from build123d import *

# Parameters (mm, degrees)
CROSSRECESS_DEPTH = 2.17
FILLET5_R         = 0.3
DRAFT1_ANGLE      = -30


with BuildPart() as part:
    # Sketch1 → Base (revolve)
    with BuildSketch(Plane.XY):
        with BuildLine():
            Line((38.1, 2), (4.5, 2))
            Line((4.5, 2), (3.1, 2))
            Line((3.1, 2), (3.1, 2.35))
            Line((3.1, 2.35), (3.1, 4))
            Line((3.1, 4), (1.376524617, 4))
            ThreePointArc((1.376524617, 4), (0.353757652, 2.115113473), (0, 0))
            Line((0, 0), (38.1, 0))
            Line((38.1, 0), (38.1, 2))
        make_face()
    revolve(axis=Axis((4.515812911, 0, 0), (-1, 0, 0)))

    # Sketch6 → CrossRecess (cut)
    with BuildSketch(Plane(origin=(0, 0, 0), x_dir=(0, 0, -1), z_dir=(1, 0, 0))):
        Polygon((0.44, 0.44), (0.44, 2.2), (-0.44, 2.2), (-0.44, 0.44), (-2.2, 0.44), (-2.2, -0.44), (-0.44, -0.44), (-0.44, -2.2), (0.44, -2.2), (0.44, -0.44), (2.2, -0.44), (2.2, 0.44), align=None)
    extrude(amount=CROSSRECESS_DEPTH, mode=Mode.SUBTRACT)

    # Fillet5
    fillet5_edges = [part.edges().sort_by_distance(p)[0] for p in [
        (1.099926585, 0.44, 0.44),
        (1.099926585, -0.44, 0.44),
        (1.099926585, -0.44, -0.44),
        (1.099926585, 0.44, -0.44),
    ]]
    fillet(fillet5_edges, radius=FILLET5_R)

    # Draft1
    draft1_faces = [part.faces().sort_by_distance(p)[0] for p in [
        (1.27944778, -2.2, 0),
        (1.27944778, 0, -2.2),
        (1.27944778, 0, 2.2),
        (1.27944778, 2.2, 0),
    ]]
    draft(draft1_faces, Plane(origin=(0, 0, 0), x_dir=(0, 0, 1), z_dir=(1, 0, 0)), DRAFT1_ANGLE)


solid = part.part
Model file for the job. Use its own axes, mm. A direction names the side the tool comes from. Give positions to 0.01 mm unless a question says otherwise; leave off trailing zeros. Loops run counter-clockwise (first coordinate to the right, second up) from the corner with the lowest first, then second, coordinate; pieces in that order, holes last. Notation, with made-up numbers: (64, 5.5) -> (72, 5.5) arc R35 cw to (72, 40.5) -> close; hole circle Ø6 at (53.5, -25.5). An arc over 180 degrees is marked (long way). Use a Markdown table: item, result. Add a question column.
(1) Slice it at C-C on x = 18.5. List the corners of the cut face in (y, z).
(2) Slice it at D-D on z = 3.5. List the corners of the cut face in (x, y).
(3) Mould opens along Z. For faces 1 (the flat face through (1, -1, -0.44)), 2 (the cylindrical face through (20, 0, 2)), 3 (the flat face through (3.1, 2, 1)) say: +Z half, -Z half, draft (parallel to the pull), parting line (faces both ways), or undercut.
(4) Slice it at A-A on z = 0. List the corners of the cut face in (x, y).
(5) Tool access for faces 4 (the cylindrical face through (2.226, -0.867, 3.905)), 5 (the flat face through (1, 1, 0.44)): list every direction of +Z, -Z, +X, -X, +Y, -Y with a clear straight run to the whole face (end or side of a thin tool).
(6) Drop flat-ended pins along their axis: pin 1 Ø1.4 at (x, y) = (0.5, 1.5) entering from -Z; pin 2 Ø4 at (x, z) = (26.5, -2) entering from +Y; pin 3 Ø1 at (y, z) = (0.5, -2) entering from -X. Give the stop position or say it passes through.
(7) Wall check: line 1 along X through (y, z) = (-0.25, 0); line 2 along X through (y, z) = (3.25, -1.75); line 3 along Z through (x, y) = (31.5, 0.25). Give the ranges that are in metal, low to high.
Filled sheet:
| question | item | result |
|---|---|---|
| 1 | outline | circle Ø4 at (0, 0) |
| 2 | outline | (1.38, -1.94) -> (3.1, -1.94) -> (3.1, 1.94) -> (1.38, 1.94) arc R5.48 ccw to start |
| 3 | face 1 | undercut |
| 3 | face 2 | parting line |
| 3 | face 3 | draft |
| 4 | outline | (0.32, -2.02) arc R6.5 ccw to (1.38, -4) -> (3.1, -4) -> (3.1, -2) -> (38.1, -2) -> (38.1, 2) -> (3.1, 2) -> (3.1, 4) -> (1.38, 4) arc R6.5 ccw to (0.32, 2.02) -> (2.17, 0.95) -> (2.17, -0.95) -> close |
| 5 | face 4 | +X, -X |
| 5 | face 5 | -X |
| 6 | pin 1 | z = -3.49 |
| 6 | pin 2 | y = 2 |
| 6 | pin 3 | x = 0.19 |
| 7 | line 1 | 2.17 to 38.1 |
| 7 | line 2 | 1.15 to 3.1 |
| 7 | line 3 | -1.98 to 1.98 |
